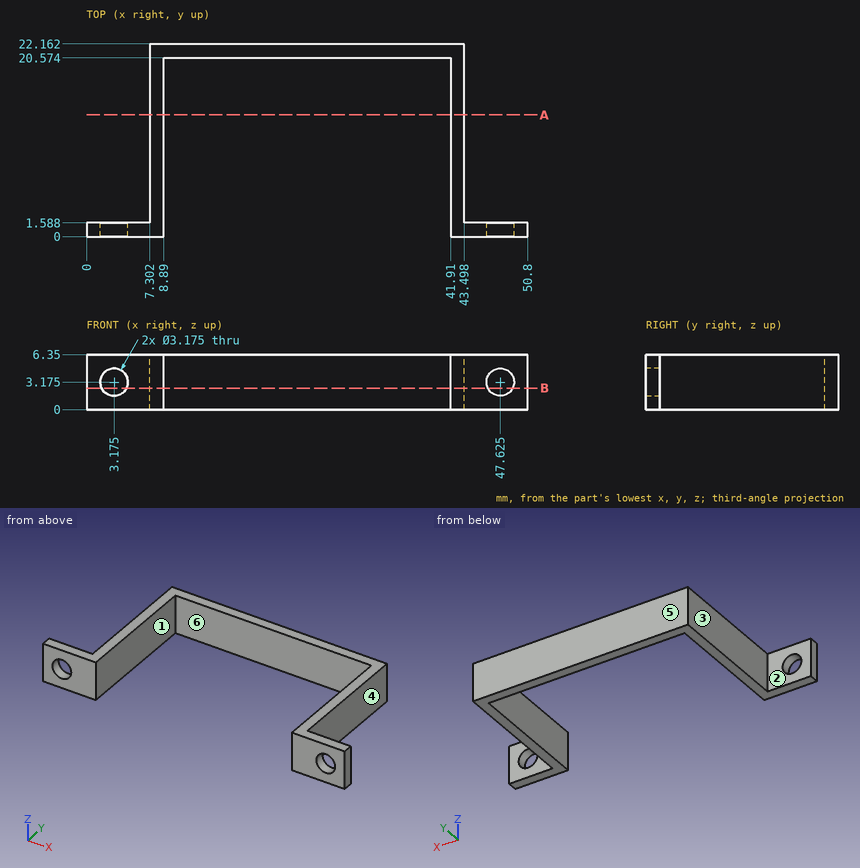
Source: three-view drawing plus pictorial views. Frame: mm from the lowest corner of the part. A direction names the side the tool comes from. Give positions to 0.01 mm unless a question says otherwise; leave off trailing zeros. Loops run counter-clockwise (first coordinate to the right, second up) from the corner with the lowest first, then second, coordinate; pieces in that order, holes last. Notation, with made-up numbers: (56.5, 16.25) -> (112.5, 16.25) arc R20 cw to (112.5, 29.25) -> close; hole circle Ø10 at (83, 79). An arc over 180 degrees is marked (long way). Put each result on its own line as item: value. Start each with the question number.
1) Reachability of the marked faces 5 and 6 from +Z, -Z, +X, -X, +Y, -Y: full face, straight path, thin tool, end or side. Return the list, or none.
2) Material intervals for probe 1 along X at (y, z) = (5.25, 4.25); probe 2 along Y at (x, z) = (9.5, 1.75) (1 decimal); probe 3 along Y at (x, z) = (3, 1), sorted ascending.
3) Contact query for flat-ended pins moving along their axis: P1, Ø2.5, axis at x = 47.625, z = 3.175, coming from the +Y side; P2, Ø3, axis at x = 27, z = 4.5, coming from the -Y side; P3, Ø1.9, axis at y = 10, z = 4, coming from the -X side; P4, Ø1.9, axis at x = 3, z = 4, coming from the +Y side. Output: stop coordinate, or through.
4) Cut plane A-A (y = 14). Return loops of the section in (x, z).
5) Cut plane B-B (z = 2.5). Return loops of the section in (x, y) (1 decimal), then the cut area to 3 significant figures.
6) Draft query along X for the marked faces 1, 2, 3 and 4. Return one class per face: released by +X, released by -X, zero draft, split by the parting line, or undercut.
Results are:
1. face 5: +Z, -Z, +X, -X, +Y
1. face 6: +Z, -Z, -Y
2. probe 1: x = 7.3 to 8.89, 41.91 to 43.5
2. probe 2: y = 20.6 to 22.2
2. probe 3: y = 0 to 1.59
3. P1: passes through
3. P2: stops at y = 20.57
3. P3: stops at x = 7.3
3. P4: stops at y = 1.59
4. outline: (7.3, 0) -> (8.89, 0) -> (8.89, 6.35) -> (7.3, 6.35) -> close; (41.91, 0) -> (43.5, 0) -> (43.5, 6.35) -> (41.91, 6.35) -> close
5. outline: (0, 0) -> (1.7, 0) -> (1.7, 1.6) -> (0, 1.6) -> close; (4.6, 0) -> (8.9, 0) -> (8.9, 20.6) -> (41.9, 20.6) -> (41.9, 0) -> (46.2, 0) -> (46.2, 1.6) -> (43.5, 1.6) -> (43.5, 22.2) -> (7.3, 22.2) -> (7.3, 1.6) -> (4.6, 1.6) -> close; (49.1, 0) -> (50.8, 0) -> (50.8, 1.6) -> (49.1, 1.6) -> close
5. area: 137 mm2
6. face 1: undercut
6. face 2: zero draft
6. face 3: released by -X
6. face 4: released by +X
